```python
from build123d import *

# Parameters (mm, degrees)
SKETCH1_R           = 0.75
BOSS_EXTRUDE1_DEPTH = 3


with BuildPart() as part:
    # Sketch1 → Boss-Extrude1 (new body)
    with BuildSketch(Plane.XY):
        with BuildLine():
            ThreePointArc((0, 27.2), (19.233304448, 19.233304448), (27.2, 0))
            ThreePointArc((27.2, 0), (-13.088306987, -23.843997572), (-14.60413384, 22.946879413))
            ThreePointArc((-14.60413384, 22.946879413), (-14.021368524, 25.569928133), (-16.644417244, 26.152693449))
            ThreePointArc((-16.644417244, 26.152693449), (8.667943905, -29.763513711), (0, 31))
            ThreePointArc((0, 31), (-1.9, 29.1), (0, 27.2))
        make_face()
        with Locations((-15.624275542, 24.549786431)):
            Circle(SKETCH1_R, mode=Mode.SUBTRACT)
        with Locations((0, 29.1)):
            Circle(SKETCH1_R, mode=Mode.SUBTRACT)
    extrude(amount=BOSS_EXTRUDE1_DEPTH)


solid = part.part
```
Geometry: final body of the model. Coordinates: model frame, mm. Give positions to 0.01 mm unless a question says otherwise; leave off trailing zeros. Order: outer loops, then holes, each group sorted by start corner. A loop starts at its lowest first (then second) coordinate and runs counter-clockwise, first axis right, second up. Notation, with made-up numbers: (54, -3.75) -> (62, -3.75) arc R24 ccw to (62, 29.25) -> close; hole circle Ø4 at (80, -1.75). An arc over 180 degrees is marked (long way). Write each question's results on one line, items separated by ' | '. Start each with the question number.
1) Draft query along Y for faces 1 (the cylindrical face through (7.47, -30.086, 1.479)), 2 (the flat face through (11.3, -25.1, 0)), 3 (the cylindrical face through (-0.098, 29.844, 1.479)), 4 (the cylindrical face through (-16.219, 24.093, 1.479)). Return one class per face: pulls with the +Y half, pulls with the -Y half, needs draft (parallel to the pull), parting line crosses it, or undercut.
2) Section D-D (x = -12). Return loops of the section in (y, z), then the cut area to 3 significant figures.
3) First-contact query: pin 1 (1.5 mm diameter, centred on x = 13.5, z = 1.5, fed in from -Y). Flat tip, straight axial feed; report the tip coordinate or a pass-through.
4) Section C-C (z = 2.1). Return loops of the section in (x, y), then the cut area to 3 significant figures.
5) Line query: line 1 (Y direction, x = 0, z = 1.1); line 2 (X direction, y = 19.5, z = 1.45); line 3 (X direction, y = 13, z = 2.2). Output: solid intervals per line, ascending. Write a range as from..to.
6) Section B-B (x = -21.5). Return loops of the section in (y, z).
7) Section A-A (y = 10). Return loops of the section in (x, z), then the cut area to 3 significant figures.
Calculated:
1) face 1: parting line crosses it | face 2: needs draft | face 3: undercut | face 4: undercut
2) outline: (-28.58, 0) -> (-24.41, 0) -> (-24.41, 3) -> (-28.58, 3) -> close | area: 12.5 mm2
3) pin 1: y = -28.26
4) outline: (-16.64, 26.15) arc R31 ccw (long way) to (0, 31) arc R1.9 ccw to (0, 27.2) arc R27.2 cw (long way) to (-14.6, 22.95) arc R1.9 ccw to start; hole circle Ø1.5 at (-15.62, 24.55); hole circle Ø1.5 at (0, 29.1) | area: 640 mm2
5) line 1: -31..-27.2, 27.2..28.35, 29.85..31 | line 2: -24.1..-18.96, 18.96..24.1 | line 3: -28.14..-23.89, 23.89..28.14
6) outline: (-22.33, 0) -> (-16.66, 0) -> (-16.66, 3) -> (-22.33, 3) -> close; (16.66, 0) -> (22.33, 0) -> (22.33, 3) -> (16.66, 3) -> close
7) outline: (-29.34, 0) -> (-25.3, 0) -> (-25.3, 3) -> (-29.34, 3) -> close; (25.3, 0) -> (29.34, 0) -> (29.34, 3) -> (25.3, 3) -> close | area: 24.3 mm2
